For this review, take the finished solid that the model builds, in its own axes (mm). A direction names the side the tool comes from. Give positions to 0.01 mm unless a question says otherwise; leave off trailing zeros. Order: outer loops, then holes, each group sorted by start corner. A loop starts at its lowest first (then second) coordinate and runs counter-clockwise, first axis right, second up. Notation, with made-up numbers: (71.5, -39.5) - (108.5, -39.5) arc R30 cw to (108.5, -9.5) - close; hole circle Ø3 at (-6.75, 16.5). An arc over 180 degrees is marked (long way). Use a Markdown table: item, result. Add a question column.
1) Machinability: for faces 1 (the face through (683.86, -0.11, 486.69)), 2 (the face through (-287.556, -0.105, 380.239)), which of the approach directions +Z, -Z, +X, -X, +Y, -Y give a long, thin tool a straight path to every point of the face, cutting with its end or side? Answer none if there is none.
2) We need section C-C on y = 0. Give the number of separate pieces and of enclosed holes in the cut face, then the cut area to 3 significant figures.
3) Mouldability with a two-part tool opening along Z and no side actions: class faces 3 (the face through (718.998, -0.105, 405.896)), 4 (the face through (277, -7.5, 273)), 5 (the face through (-266.185, -0.105, -34.561)), 6 (the face through (-251.13, -0.11, 203.36)) as released by +Z, released by -Z, zero draft, split by the parting line, or undercut.
4) We need section A-A on z = 187.5. Write out the cut boundary in (x, y).
5) Wall thickness on L1, parallel to X at y = -5.25, z = 333; L2, parallel to Z at x = 102.5, y = 2.75; L3, parallel to X at y = -5, z = 97: over which ranges is each line inside the solid? List them lowest first.
6) We need section B-B on x = -26. Write out the cut boundary in (y, z).
7) Clearance check with flat-ended pins moving along their axes: P1, Ø1.5, axis at y = 5.5, z = 149.5, coming from the -X side; P2, Ø9, axis at x = 636.32, z = 394.43, coming from the +Y side; P3, Ø4.5, axis at y = 2, z = 490, coming from the +X side; P4, Ø4.5, axis at y = -2, z = 489.5, coming from the -X side. State where each tip first meets the part, or that it passes through.
```python
from build123d import *

# Parameters (mm, degrees)
F0_R     = 10
F0_R_2   = 20
F0_R_3   = 4
F1_DEPTH = 7.5


with BuildPart() as f1:
    # F0 (on Front) → F1 (new body, symmetric)
    with BuildSketch(Plane.XZ):
        with BuildLine():
            ThreePointArc((-275.56228, -20.548175), (-265.997427, -34.715036), (-250.213495, -41.276581))
            Line((-250.213495, -41.276581), (207.372435, -88.341603))
            ThreePointArc((207.372435, -88.341603), (253.099825, -83.652204), (293.182151, -61.149053))
            Line((293.182151, -61.149053), (726.156602, 315.743114))
            ThreePointArc((726.156602, 315.743114), (736.385608, 331.867799), (736.13455, 350.961647))
            Line((736.13455, 350.961647), (701.375468, 462.389844))
            ThreePointArc((701.375468, 462.389844), (683.514294, 486.942452), (654.636412, 496.31902))
            Line((654.636412, 496.31902), (-79.706343, 496.31902))
            Line((-79.706343, 496.31902), (-79.706343, 481.31902))
            Line((-79.706343, 481.31902), (-94.706343, 481.31902))
            Line((-94.706343, 481.31902), (-94.706343, 496.31902))
            Line((-94.706343, 496.31902), (-134.706343, 496.31902))
            Line((-134.706343, 496.31902), (-134.706343, 481.31902))
            Line((-134.706343, 481.31902), (-149.706343, 481.31902))
            Line((-149.706343, 481.31902), (-149.706343, 496.31902))
            Line((-149.706343, 496.31902), (-189.706343, 496.31902))
            Line((-189.706343, 496.31902), (-189.706343, 481.31902))
            Line((-189.706343, 481.31902), (-204.706343, 481.31902))
            Line((-204.706343, 481.31902), (-204.706343, 496.31902))
            Line((-204.706343, 496.31902), (-244.706343, 496.31902))
            Line((-244.706343, 496.31902), (-244.706343, 481.31902))
            Line((-244.706343, 481.31902), (-259.706343, 481.31902))
            Line((-259.706343, 481.31902), (-259.706343, 496.31902))
            Line((-259.706343, 496.31902), (-299.706343, 496.31902))
            Line((-299.706343, 496.31902), (-299.706343, 481.31902))
            Line((-299.706343, 481.31902), (-314.706343, 481.31902))
            Line((-314.706343, 481.31902), (-314.706343, 496.31902))
            Line((-314.706343, 496.31902), (-354.706343, 496.31902))
            Line((-354.706343, 496.31902), (-354.706343, 481.31902))
            Line((-354.706343, 481.31902), (-369.706343, 481.31902))
            Line((-369.706343, 481.31902), (-369.706343, 496.31902))
            Line((-369.706343, 496.31902), (-395.363588, 496.31902))
            ThreePointArc((-395.363588, 496.31902), (-419.913193, 483.901328), (-424.456906, 456.767643))
            Line((-424.456906, 456.767643), (-275.56228, -20.548175))
        make_face()
        with Locations((-232.248772, -13.546013)):
            Circle(F0_R, mode=Mode.SUBTRACT)
        with BuildLine():
            Line((-208.053878, 65.265342), (-295.432418, 345.377263))
            ThreePointArc((-295.432418, 345.377263), (-287.23091, 380.65043), (-254.581922, 396.31902))
            Line((-254.581922, 396.31902), (193.565616, 396.31902))
            ThreePointArc((193.565616, 396.31902), (225.221488, 385.930207), (244.565755, 358.804187))
            Line((244.565755, 358.804187), (319.042257, 120.052707))
            ThreePointArc((319.042257, 120.052707), (319.750596, 92.90088), (306.101749, 69.418282))
            Line((306.101749, 69.418282), (238.217744, 10.327151))
            ThreePointArc((238.217744, 10.327151), (223.342417, 1.911302), (206.358638, 0))
            Line((206.358638, 0), (-168.811503, 33.604402))
            ThreePointArc((-168.811503, 33.604402), (-193.239091, 43.477544), (-208.053878, 65.265342))
        make_face(mode=Mode.SUBTRACT)
        with Locations((230.366445, -43.535308)):
            Circle(F0_R_2, mode=Mode.SUBTRACT)
        with Locations((363.418511, 151.143091)):
            Circle(F0_R_3, mode=Mode.SUBTRACT)
        with Locations((430.203208, 166.843278)):
            Circle(F0_R_3, mode=Mode.SUBTRACT)
        with Locations((-397.907798, 435.702402)):
            Circle(F0_R_3, mode=Mode.SUBTRACT)
        with Locations((-407.3259, 464.338549)):
            Circle(F0_R_3, mode=Mode.SUBTRACT)
        with Locations((-388.363458, 480.715226)):
            Circle(F0_R_3, mode=Mode.SUBTRACT)
        with BuildLine():
            ThreePointArc((-348.862556, 424.598233), (-363.862556, 439.598233), (-348.862556, 454.598233))
            Line((-348.862556, 454.598233), (-78.862556, 454.598233))
            ThreePointArc((-78.862556, 454.598233), (-63.862556, 439.598233), (-78.862556, 424.598233))
            Line((-78.862556, 424.598233), (-348.862556, 424.598233))
        make_face(mode=Mode.SUBTRACT)
        with Locations((-11.091434, 477.31902)):
            Circle(F0_R_3, mode=Mode.SUBTRACT)
        with Locations((46.90848, 477.31902)):
            Circle(F0_R_3, mode=Mode.SUBTRACT)
        with Locations((104.90848, 477.31902)):
            Circle(F0_R_3, mode=Mode.SUBTRACT)
        with Locations((324.477992, 258.924084)):
            Circle(F0_R_3, mode=Mode.SUBTRACT)
        with Locations((391.262689, 274.624271)):
            Circle(F0_R_3, mode=Mode.SUBTRACT)
        with BuildLine():
            Line((437.654594, 243.525634), (399.05919, 367.25204))
            ThreePointArc((399.05919, 367.25204), (402.398442, 387.193047), (420.440365, 396.31902))
            Line((420.440365, 396.31902), (579.801329, 396.31902))
            ThreePointArc((579.801329, 396.31902), (590.691559, 392.745068), (597.34636, 383.413194))
            Line((597.34636, 383.413194), (608.896369, 346.386995))
            ThreePointArc((608.896369, 346.386995), (609.023108, 336.747995), (603.859278, 328.607894))
            Line((603.859278, 328.607894), (489.3056, 228.892116))
            ThreePointArc((489.3056, 228.892116), (459.519244, 222.228502), (437.654594, 243.525634))
        make_face(mode=Mode.SUBTRACT)
        with Locations((648.709043, 338.435646)):
            Circle(F0_R_3, mode=Mode.SUBTRACT)
        with Locations((694.243557, 339.484597)):
            Circle(F0_R_3, mode=Mode.SUBTRACT)
        with Locations((288.051486, 357.594401)):
            Circle(F0_R_3, mode=Mode.SUBTRACT)
        with Locations((354.836183, 373.294587)):
            Circle(F0_R_3, mode=Mode.SUBTRACT)
        with Locations((162.90848, 477.31902)):
            Circle(F0_R_3, mode=Mode.SUBTRACT)
        with Locations((636.319377, 394.431325)):
            Circle(F0_R_3, mode=Mode.SUBTRACT)
        with Locations((681.85389, 395.480275)):
            Circle(F0_R_3, mode=Mode.SUBTRACT)
        with Locations((624.388255, 455.463381)):
            Circle(F0_R_3, mode=Mode.SUBTRACT)
        with Locations((669.922769, 456.512332)):
            Circle(F0_R_3, mode=Mode.SUBTRACT)
    extrude(amount=F1_DEPTH, both=True)


solid = f1.part
```
Checked values:
| question | item | result |
|---|---|---|
| 1 | face 1 | +Z, +X, +Y, -Y |
| 1 | face 2 | +Y, -Y |
| 2 | separate pieces | 1 |
| 2 | enclosed holes | 24 |
| 2 | area | 279,000 mm² |
| 3 | face 3 | released by +Z |
| 3 | face 4 | zero draft |
| 3 | face 5 | released by -Z |
| 3 | face 6 | undercut |
| 4 | outline | (-340.46, -7.5) - (-246.18, -7.5) - (-246.18, 7.5) - (-340.46, 7.5) - close; (298, -7.5) - (578.83, -7.5) - (578.83, 7.5) - (298, 7.5) - close |
| 5 | L1 | -385.85 to -291.57, 252.62 to 409.74, 607.45 to 736.69 |
| 5 | L2 | -77.55 to 9.3, 396.32 to 474.13, 480.51 to 496.32 |
| 5 | L3 | -312.23 to -217.95, 320.62 to 474.86 |
| 6 | outline | (-7.5, -64.34) - (7.5, -64.34) - (7.5, 20.81) - (-7.5, 20.81) - close; (-7.5, 396.32) - (7.5, 396.32) - (7.5, 496.32) - (-7.5, 496.32) - close |
| 7 | P1 | x = -328.84 |
| 7 | P2 | y = 7.5 |
| 7 | P3 | x = 682.37 |
| 7 | P4 | x = -417.06 |
